```python
from build123d import *

# Parameters (mm, degrees)
SKETCH1_W               = 20.5
SKETCH1_H               = 8
BOSS_EXTRUDE1_DEPTH     = 3
CUT_EXTRUDE1_DEPTH      = 23.209232315
CUT_EXTRUDE1_DEPTH_BACK = 23.209232315
CUT_EXTRUDE2_DEPTH      = 23.209232315
CUT_EXTRUDE2_DEPTH_BACK = 23.209232315
SKETCH4_R               = 1.75
CUT_EXTRUDE3_DEPTH      = 0.4
SKETCH5_W               = 8
SKETCH5_H               = 1.2
BOSS_EXTRUDE2_DEPTH     = 2
FILLET1_R               = 4


with BuildPart() as part:
    # Sketch1 → Boss-Extrude1 (new body)
    with BuildSketch(Plane(origin=(0, 0, 0), x_dir=(1, 0, 0), z_dir=(0, 1, 0))):
        with Locations((10.25, 4)):
            Rectangle(SKETCH1_W, SKETCH1_H)
    extrude(amount=BOSS_EXTRUDE1_DEPTH)

    # Sketch2 → Cut-Extrude1 (cut, two sides: drawn at the far end of the back side and taken through both)
    with BuildSketch(Plane.XY.offset(-CUT_EXTRUDE1_DEPTH_BACK)):
        Polygon((0, 0), (0.6, 3), (0, 3), align=None)
        Polygon((20.5, 0), (19.9, 3), (20.5, 3), align=None)
    extrude(amount=CUT_EXTRUDE1_DEPTH + CUT_EXTRUDE1_DEPTH_BACK, mode=Mode.SUBTRACT)

    # Sketch3 → Cut-Extrude2 (cut, two sides: drawn at the far end of the back side and taken through both)
    with BuildSketch(Plane(origin=(0, 0, 0), x_dir=(0, 0, -1), z_dir=(1, 0, 0)).offset(-CUT_EXTRUDE2_DEPTH_BACK)):
        Polygon((0, 0), (0.6, 3), (0, 3), align=None)
        Polygon((8, 3), (7.4, 3), (8, 0), align=None)
    extrude(amount=CUT_EXTRUDE2_DEPTH + CUT_EXTRUDE2_DEPTH_BACK, mode=Mode.SUBTRACT)

    # Sketch4 → Cut-Extrude3 (cut)
    with BuildSketch(Plane.XZ):
        with Locations(Location((10.25000125, -3.75, 0), (0, 0, 270))):
            Circle(SKETCH4_R)
    extrude(amount=-CUT_EXTRUDE3_DEPTH, mode=Mode.SUBTRACT)

    # Sketch5 → Boss-Extrude2 (add)
    with BuildSketch(Plane.XZ):
        with Locations((10.250011, -7.4)):
            Rectangle(SKETCH5_W, SKETCH5_H)
    extrude(amount=BOSS_EXTRUDE2_DEPTH)

    # Fillet1
    # the kernel refuses this fillet: 4 mm, written as the material it takes off along each edge
    with BuildSketch(Plane(origin=(14.250011, -2, -16.660254038), x_dir=(0, 1, 0), z_dir=(0, 0, 1)), Plane(origin=(6.250011, -2, 1.860254038), x_dir=(0, 1, 0), z_dir=(0, 0, -1))) as fillet1_piece_1:
        with BuildLine():
            CenterArc((4, 3.464101615), FILLET1_R, 180, 60)
            Line((0, 3.464101615), (-0.08, 3.464101615))
            Line((-0.08, 3.464101615), (-0.08, 0))
            Line((-0.08, 0), (0, -0.08))
            ThreePointArc((0, -0.08), (1, -0.08), (1.96, -0.069282032))
            Line((1.96, -0.069282032), (2, 0))
        make_face()
    extrude(amount=18.520508076, mode=Mode.SUBTRACT)


solid = part.part
```
Source: CAD feature listing. Evaluate the final solid. Frame: model axes, mm. A direction names the side the tool comes from. Coordinates: 2 decimals unless noted, no trailing zeros. Loops run counter-clockwise (first coordinate to the right, second up) from the corner with the lowest first, then second, coordinate; pieces in that order, holes last. Notation, with made-up numbers: M 60.25,52 L 104.25,52 A16 cw 104.25,67 Z; hole C 37.25,87 d6. An arc over 180 degrees is marked long. Use a Markdown table: item, result. Add a question column.
Q1. Material intervals for L1, parallel to Y at x = 9.5, z = -3.75; L2, parallel to Y at x = 3, z = -1.75; L3, parallel to X at y = 0.3, z = -3.75, sorted ascending.
Q2. First-contact query: pin 1 (1.5 mm diameter, centred on x = 13, y = -1, fed in from +Z); pin 2 (2.5 mm diameter, centred on x = 11.5, z = -3, fed in from -Y); pin 3 (1 mm diameter, centred on x = 10, z = -4.5, fed in from -Y). Flat tips, straight axial feed; report the tip coordinate or a pass-through.
Q3. Section query D-D, the plane z = -5. Return loops of the section in (x, y).
Q4. Section query B-B, the plane x = 13.5. Return loops of the section in (y, z).
Q5. Access query for faces 5 (the flat face through (10, -1, -6.8)), 6 (the flat face through (10.1, 1.5, -7.7)). Directions: +Z, -Z, +X, -X, +Y, -Y. A direction counts if a zero-diameter tool reaches every point of the face in a straight line with its end or side. Return the directions, or none.
Q6. Draft query along X for faces 1 (the flat face through (10, 0.4, -4)), 2 (the cylindrical face through (12.76, -1.48, -7.41)), 3 (the cylindrical face through (8.54, 0.2, -3.37)), 4 (the flat face through (10.1, 1.5, -0.3)). Return one class per face: pulls with the +X half, pulls with the -X half, needs draft (parallel to the pull), parting line crosses it, or undercut.
Q7. Section query C-C, the plane y = 0.7. Return loops of the section in (x, z), and give its area (3 significant figures).
Q8. Section query A-A, the plane z = -3.75. Return loops of the section in (x, y), and give its area (3 significant figures).
Result:
| question | item | result |
|---|---|---|
| 1 | L1 | y = 0.4 to 3 |
| 1 | L2 | y = 0 to 3 |
| 1 | L3 | x = 0.06 to 8.5, 12 to 20.44 |
| 2 | pin 1 | stops at z = -6.8 |
| 2 | pin 2 | stops at y = 0 |
| 2 | pin 3 | stops at y = 0.4 |
| 3 | outline | M 0,0 L 9.03,0 L 9.03,0.4 L 11.47,0.4 L 11.47,0 L 20.5,0 L 19.9,3 L 0.6,3 Z |
| 4 | outline | M -0.94,-8 L 0,-8 L 3,-7.4 L 3,-0.6 L 0,0 L 0,-6.8 L -0.94,-6.8 Z |
| 5 | face 5 | +Z, +X, -X, -Y |
| 5 | face 6 | -Z, +X, -X, +Y |
| 6 | face 1 | undercut |
| 6 | face 2 | pulls with the +X half |
| 6 | face 3 | undercut |
| 6 | face 4 | needs draft |
| 7 | outline | M 0.14,-7.86 L 20.36,-7.86 L 20.36,-0.14 L 0.14,-0.14 Z |
| 7 | area | 156 mm2 |
| 8 | outline | M 0,0 L 8.5,0 L 8.5,0.4 L 12,0.4 L 12,0 L 20.5,0 L 19.9,3 L 0.6,3 Z |
| 8 | area | 58.3 mm2 |
